Could you check a few things on this drawing? It's one solid part, dimensions in mm from its lowest x, y, z. A direction names the side the tool comes from. Round coordinates to 2 decimals unless told otherwise and drop trailing zeros. Order: outer loops, then holes, each group sorted by start corner. A loop starts at its lowest first (then second) coordinate and runs counter-clockwise, first axis right, second up. Notation, with made-up numbers: (3.25, 76) -> (28.25, 76) arc R24 ccw to (28.25, 105) -> close; hole circle Ø9 at (58.5, 67.25). An arc over 180 degrees is marked (long way). Use a Markdown table: item, result. Add a question column.
(1) I'm going to push flat-ended pins straight in: P1, Ø21, axis at y = 35, z = 35, coming from the -X side; P2, Ø20, axis at x = 58.5, z = 57.5, coming from the +Y side; P3, Ø1.5, axis at x = 10, z = 37.5, coming from the -Y side; P4, Ø9, axis at x = 44.5, z = 38.5, coming from the -Y side. Where does each tip first touch, or does it pass through?
(2) If I drill on probe 1 along X at (y, z) = (57.5, 18); probe 2 along Y at (x, z) = (70, 35); probe 3 along Y at (x, z) = (52, 62.5), over which ranges is the centre line in solid material (lowest first)?
(3) I want a section at B-B, the plane z = 49. Please give me the cut outline in (x, y).
(4) I want a section at A-A, the plane y = 38. Please give me the cut outline in (x, z).
(5) On a 3-axis mill with a long thin cutter (end or side, diameter ignored), from which of +Z, -Z, +X, -X, +Y, -Y can I reach the whole of each face in a straight line? I mean the marked faces 4, 5, 6, 7 and 8. Say none if no direction works.
(6) Thinking about a two-plate mould opening in X: for the marked faces 1, 2 and 3, which applies, pulls with the +X half, pulls with the -X half, needs draft (parallel to the pull), parting line crosses it, or undercut?
(7) I want a section at C-C, the plane x = 71. Please give me the cut outline in (y, z).
(8) I want a section at D-D, the plane z = 58. Please give me the cut outline in (x, y), then the cut area to 3 significant figures.
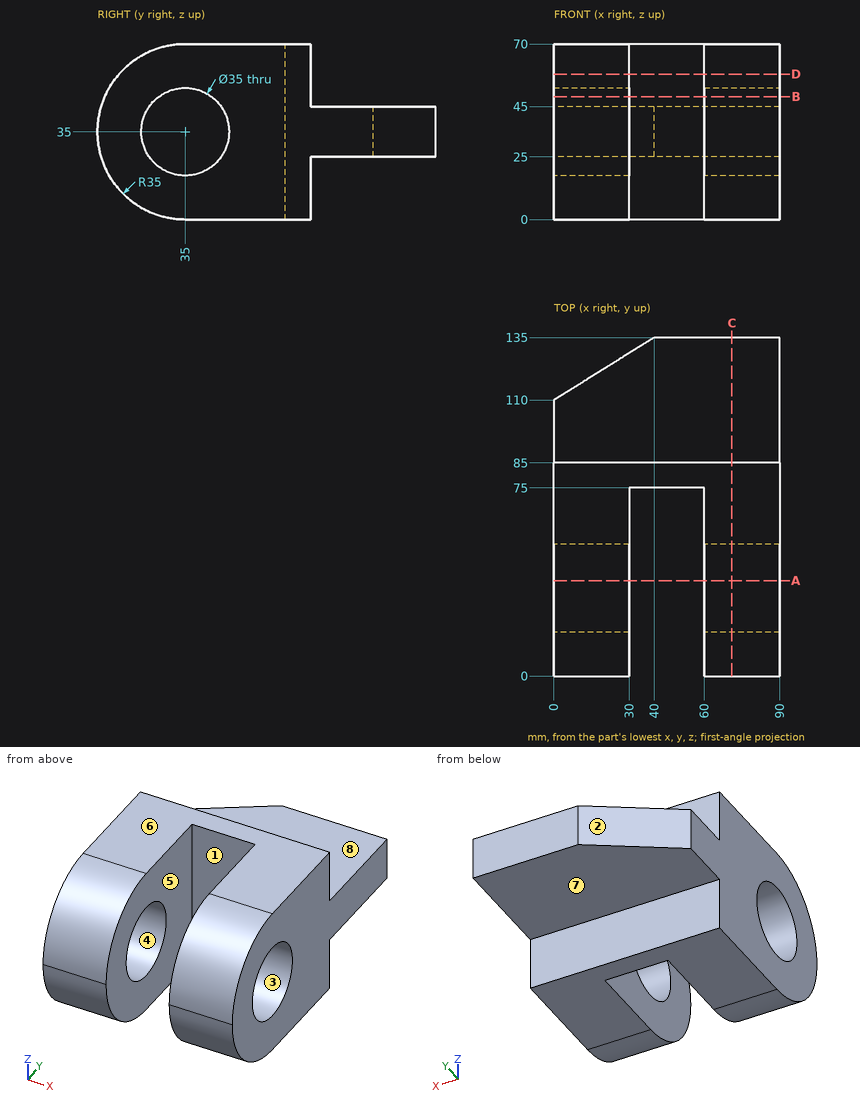
Taken from the geometry:
| question | item | result |
|---|---|---|
| 1 | P1 | passes through |
| 1 | P2 | stops at y = 85 |
| 1 | P3 | stops at y = 0.04 |
| 1 | P4 | stops at y = 75 |
| 2 | probe 1 | x = 0 to 30, 60 to 90 |
| 2 | probe 2 | y = 0 to 17.5, 52.5 to 135 |
| 2 | probe 3 | y = 75 to 85 |
| 3 | outline | (0, 2.92) -> (30, 2.92) -> (30, 24.5) -> (0, 24.5) -> close; (0, 45.5) -> (30, 45.5) -> (30, 75) -> (60, 75) -> (60, 45.5) -> (90, 45.5) -> (90, 85) -> (0, 85) -> close; (60, 2.92) -> (90, 2.92) -> (90, 24.5) -> (60, 24.5) -> close |
| 4 | outline | (0, 0) -> (30, 0) -> (30, 17.76) -> (0, 17.76) -> close; (0, 52.24) -> (30, 52.24) -> (30, 70) -> (0, 70) -> close; (60, 0) -> (90, 0) -> (90, 17.76) -> (60, 17.76) -> close; (60, 52.24) -> (90, 52.24) -> (90, 70) -> (60, 70) -> close |
| 5 | face 4 | +X, -X |
| 5 | face 5 | +Z, -Z, -Y |
| 5 | face 6 | +Z, +X, -X, +Y, -Y |
| 5 | face 7 | -Z, +X, -X, +Y |
| 5 | face 8 | +Z, +X, -X, +Y |
| 6 | face 1 | undercut |
| 6 | face 2 | pulls with the -X half |
| 6 | face 3 | needs draft |
| 7 | outline | (35, 0) -> (85, 0) -> (85, 25) -> (135, 25) -> (135, 45) -> (85, 45) -> (85, 70) -> (35, 70) arc R35 ccw to start; hole circle Ø35 at (35, 35) |
| 8 | outline | (0, 8.62) -> (30, 8.62) -> (30, 75) -> (60, 75) -> (60, 8.62) -> (90, 8.62) -> (90, 85) -> (0, 85) -> close |
| 8 | area | 4,880 mm2 |
